The model under review builds one solid part; all positions refer to its coordinate system, in mm. Face numbers are marked on the shaded views. Give positions to 0.01 mm unless a question says otherwise; leave off trailing zeros. Order: outer loops, then holes, each group sorted by start corner. A loop starts at its lowest first (then second) coordinate and runs counter-clockwise, first axis right, second up. Notation, with made-up numbers: (-33, -10) - (9, -10) arc R17 ccw to (9, 11) - close; hole circle Ø8 at (45.25, 2.25). An arc over 180 degrees is marked (long way). Write item = value, one per line. Start each with the question number.
1. We need section D-D, the plane x = 33.5. Give the boundary of the cut face in (y, z).
2. We need section A-A, the plane y = 2.25. Give the boundary of the cut face in (x, z), and give its area (3 significant figures).
3. Wall thickness on probe 1 along X at (y, z) = (1.8, -5); probe 2 along Z at (x, y) = (5, 2.85); probe 3 along X at (y, z) = (0.8, -5): over which ranges is each line inside the solid? List them lowest first.
4. For P1, Ø1.5, axis at x = 8.5, z = -14, coming from the -Y side; P2, Ø12, axis at x = 20, z = -15, coming from the +Y side; P3, Ø4.5, axis at x = 5, z = -25, coming from the +Y side, all flat-tipped, find the tip position at first contact; note any pin that passes through.
5. We need section B-B, the plane z = -15. Give the boundary of the cut face in (x, y).
6. Mouldability with a two-part tool opening along X and no side actions: class the marked faces 1, 2, 3 and 4 as pulls with the +X half, pulls with the -X half, needs draft (parallel to the pull), parting line crosses it, or undercut.
7. We need section C-C, the plane x = 16.5. Give the boundary of the cut face in (y, z).
Autodesk Inventor part; units mm, degrees
ref_plane "YZ Plane" through (0, 0, 0) normal (1, 0, 0) x (0, 1, 0)
ref_plane "XZ Plane" through (0, 0, 0) normal (0, 1, 0) x (-1, 0, 0)
ref_plane "XY Plane" through (0, 0, 0) normal (0, 0, 1) x (1, 0, 0)
sketch "Sketch1" plane through (0, 0, 0) normal (0, 1, 0) x (-1, 0, 0)
  line L0 (0, 0) -> (-40, 0)
  line L1 (-40, 0) -> (-40, -30)
  line L2 (-40, -30) -> (0, -30)
  line L3 (0, -30) -> (0, 0)
  dimension "d0" = 30
  dimension "d1" = 40
extrude "Extrusion1" add sketch "Sketch1" along normal blind 3
sketch "Sketch2" plane through (0, 3, 0) normal (0, 1, 0) x (1, 0, 0)
  circle A0 centre (20, 15) radius 13
  line L0 (0, 30) -> (0, 0)
  line L1 (0, 0) -> (40, 0)
  line L2 (8.5, 3.5) -> (31.5, 3.5)
  line L3 (31.5, 3.5) -> (31.5, 26.5)
  line L4 (31.5, 26.5) -> (8.5, 26.5)
  line L5 (8.5, 26.5) -> (8.5, 3.5)
  line L6 (40, 0) -> (40, 30)
  dimension "d4" = 20
  dimension "d5" = 26
  dimension "d25" = 15
  dimension "d29" = 23
  dimension "d30" = 23
  dimension "d31" = 3.5
  dimension "d32" = 8.5
extrude "Extrusion2" cut sketch "Sketch2" against normal blind 2.5 contours A0 L3 | L3 A0 L2 L5 L4 | L4 A0 | A0 L2 | L5 A0
sketch "Sketch3" plane through (20, 0.5, -15) normal (0, 1, 0) x (1, 0, 0)
  circle A0 centre (0, 0) radius 7.5
  point P0 (-20, -15)
  dimension "d8" = 15
extrude "Extrusion3" cut sketch "Sketch3" against normal blind 3.5
sketch "Sketch4" plane through (0, 3, 0) normal (0, 1, 0) x (1, 0, 0)
  circle A0 centre (5, 5) radius 2.5
  circle A1 centre (5, 25) radius 2.5
  circle A2 centre (35, 5) radius 2.5
  circle A3 centre (35, 25) radius 2.5
  circle A4 centre (20, 15) radius 7.5
  point P0 (0, 0)
  dimension "d11" = 5
  dimension "d12" = 5
  dimension "d13" = 5
  dimension "d14" = 5
  dimension "d15" = 15
  dimension "d16" = 15
  dimension "d17" = 15
  dimension "d18" = 15
  dimension "d19" = 10
  dimension "d20" = 10
  dimension "d21" = 10
  dimension "d22" = 10
extrude "Extrusion4" cut sketch "Sketch4" against normal blind 1.7 contours A0 | A1 | A2 | A3
chamfer "Chamfer1" distance 4 angle 45 1 edges at (40, 1.5, -30)
chamfer "Chamfer2" distance 4 angle 45 1 edges at (40, 1.5, 0)
chamfer "Chamfer3" distance 4 angle 45 1 edges at (0, 1.5, 0)
chamfer "Chamfer4" distance 4 angle 45 1 edges at (0, 1.5, -30)
sketch "Sketch5" plane through (0, 3, 0) normal (0, 1, 0) x (1, 0, 0)
  line L0 (8.5, 3.5) -> (31.5, 3.5)
  line L1 (31.5, 3.5) -> (31.5, 26.5)
  line L2 (31.5, 26.5) -> (8.5, 26.5)
  line L3 (8.5, 26.5) -> (8.5, 3.5)
  line L4 (4, 0) -> (36, 0)
  line L5 (40, 4) -> (40, 26)
  point P0 (0, 0)
  dimension "d42" = 23
  dimension "d43" = 23
  dimension "d44" = 3.5
  dimension "d45" = 8.5
extrude "Extrusion5" cut sketch "Sketch5" against normal blind 2.5
properties part number "chamber_bottom"
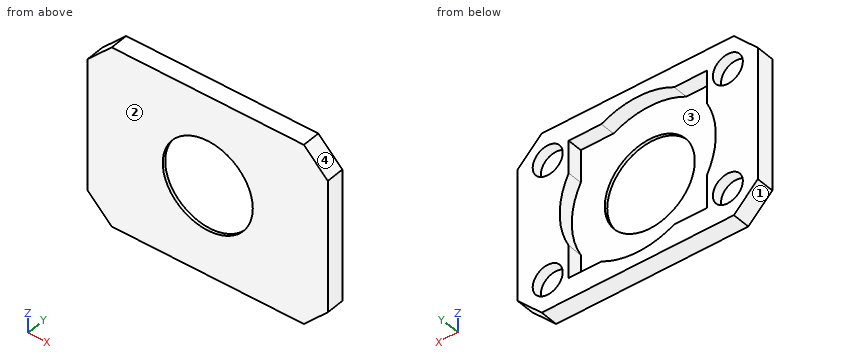
Model answer:
q1.outline = (0, -30) - (3, -30) - (3, -27) - (1.3, -27) - (1.3, -23) - (3, -23) - (3, -7) - (1.3, -7) - (1.3, -3) - (3, -3) - (3, 0) - (0, 0) - close
q2.outline = (0, -26) - (4, -30) - (36, -30) - (40, -26) - (40, -4) - (36, 0) - (4, 0) - (0, -4) - close; hole circle Ø5 at (5, -25); hole circle Ø5 at (5, -5); hole (8.5, -26.5) - (13.94, -26.5) arc R13 ccw to (26.06, -26.5) - (31.5, -26.5) - (31.5, -21.06) arc R13 ccw to (31.5, -8.94) - (31.5, -3.5) - (26.06, -3.5) arc R13 ccw to (13.94, -3.5) - (8.5, -3.5) - (8.5, -8.94) arc R13 ccw to (8.5, -21.06) - close; hole circle Ø5 at (35, -25); hole circle Ø5 at (35, -5)
q2.area = 511 mm2
q3.probe_1 = 0 to 2.5, 7.5 to 8.5, 31.5 to 32.5, 37.5 to 40
q3.probe_2 = -30 to -27.5, -22.5 to -7.5, -2.5 to 0
q3.probe_3 = 0 to 8.5, 31.5 to 40
q4.P1 = 0
q4.P2 = through
q4.P3 = 1.3
q5.outline = (0, 0) - (12.5, 0) - (12.5, 0.5) - (7, 0.5) - (7, 3) - (0, 3) - close; (27.5, 0) - (40, 0) - (40, 3) - (33, 3) - (33, 0.5) - (27.5, 0.5) - close
q6.face_1 = pulls with the -X half
q6.face_2 = needs draft
q6.face_3 = undercut
q6.face_4 = pulls with the +X half
q7.outline = (0, -30) - (3, -30) - (3, -27.52) - (0.5, -27.52) - (0.5, -21.63) - (0, -21.63) - close; (0, -8.37) - (0.5, -8.37) - (0.5, -2.48) - (3, -2.48) - (3, 0) - (0, 0) - close
